```python
from build123d import *

# Parameters (mm, degrees)
SKETCH1_R           = 4.5
SKETCH1_R_2         = 2.55
BOSS_EXTRUDE1_DEPTH = 3
SKETCH2_R           = 2.55
BOSS_EXTRUDE2_DEPTH = 4
CHAMFER1_SIZE       = 2
CUT_EXTRUDE1_DEPTH  = 32.132780152
BOSS_EXTRUDE4_DEPTH = 5
CHAMFER2_SIZE       = 1


with BuildPart() as part:
    # Sketch1 → Boss-Extrude1 (new body)
    with BuildSketch(Plane(origin=(0, 0, 0), x_dir=(1, 0, 0), z_dir=(0, 1, 0))):
        with Locations(Location((0, 0, 0), (0, 0, 270))):
            Circle(SKETCH1_R)
        with Locations(Location((0, 0, 0), (0, 0, 270))):
            Circle(SKETCH1_R_2, mode=Mode.SUBTRACT)
    extrude(amount=BOSS_EXTRUDE1_DEPTH)

    # Sketch2 → Boss-Extrude2 (add)
    with BuildSketch(Plane(origin=(0, 3, 0), x_dir=(1, 0, 0), z_dir=(0, 1, 0))):
        with BuildLine():
            Line((0, -4.5), (30, -4.5))
            Line((30, -4.5), (30, 4.5))
            Line((30, 4.5), (0, 4.5))
            ThreePointArc((0, 4.5), (-4.5, 0), (0, -4.5))
        make_face()
        with Locations(Location((0, 0, 0), (0, 0, 270))):
            Circle(SKETCH2_R, mode=Mode.SUBTRACT)
    extrude(amount=BOSS_EXTRUDE2_DEPTH)

    # Chamfer1
    # the kernel refuses this chamfer: 2 mm, written as the material it takes off along each edge
    with BuildSketch(Plane(origin=(28.666666667, 4.333333333, 3.166666667), x_dir=(-0.7071067811865475, -0.7071067811865475, 0), z_dir=(0.5773502691896256, -0.5773502691896258, 0.5773502691896258))) as chamfer1_piece_1:
        Polygon((-1.414213562, 0.816496581), (1.414213562, 0.816496581), (0, -1.632993162), align=None)
    extrude(amount=2.540341184, mode=Mode.SUBTRACT)
    with BuildSketch(Plane(origin=(28.666666667, 4.333333333, -3.166666667), x_dir=(-0.7071067811865476, -0.7071067811865475, 0), z_dir=(0.5773502691896256, -0.5773502691896258, -0.5773502691896257))) as chamfer1_piece_2:
        Polygon((-1.414213562, -0.816496581), (1.414213562, -0.816496581), (0, 1.632993162), align=None)
    extrude(amount=2.540341184, mode=Mode.SUBTRACT)
    with BuildSketch(Plane(origin=(-5.143365976, 3, 4.5), x_dir=(0, -0.027495876610586275, -0.9996219169112968), z_dir=(1, 0, 0))) as chamfer1_piece_3_section:
        Polygon((CHAMFER1_SIZE * 0.999621916911, CHAMFER1_SIZE * 0.0274958766106), (-CHAMFER1_SIZE * 0.0274958766106, CHAMFER1_SIZE * 0.999621916911), (0, 0), align=None)
    chamfer1_piece_3 = extrude(amount=40.286731952, mode=Mode.PRIVATE)
    chamfer1_piece_3 = chamfer1_piece_3 - Plane(origin=(0, 3.673505516, 0), x_dir=(0, 0, 1), z_dir=(0, -1, 0)) * Cylinder(4.5, 89, mode=Mode.PRIVATE)
    add(chamfer1_piece_3, mode=Mode.SUBTRACT)
    with BuildSketch(Plane(origin=(30, 3, 9.643365976), x_dir=(-0.9996219169112968, -0.027495876610586296, 0), z_dir=(0, 0, -1))) as chamfer1_piece_4:
        Polygon((CHAMFER1_SIZE * 0.999621916911, CHAMFER1_SIZE * 0.0274958766106), (-CHAMFER1_SIZE * 0.0274958766106, CHAMFER1_SIZE * 0.999621916911), (0, 0), align=None)
    extrude(amount=19.286731952, mode=Mode.SUBTRACT)
    with BuildSketch(Plane(origin=(30, -2.143365976, 4.5), x_dir=(-0.9996219169112968, 0, 0.02749587661058651), z_dir=(0, 1, 0))) as chamfer1_piece_5:
        Polygon((CHAMFER1_SIZE * 0.999621916911, -CHAMFER1_SIZE * 0.0274958766106), (-CHAMFER1_SIZE * 0.0274958766106, -CHAMFER1_SIZE * 0.999621916911), (0, 0), align=None)
    extrude(amount=14.286731952, mode=Mode.SUBTRACT)
    with BuildSketch(Plane(origin=(35.143365976, 3, -4.5), x_dir=(0, -0.027495876610586275, 0.9996219169112968), z_dir=(-1, 0, 0))) as chamfer1_piece_6_section:
        Polygon((CHAMFER1_SIZE * 0.999621916911, CHAMFER1_SIZE * 0.0274958766106), (-CHAMFER1_SIZE * 0.0274958766106, CHAMFER1_SIZE * 0.999621916911), (0, 0), align=None)
    chamfer1_piece_6 = extrude(amount=40.286731952, mode=Mode.PRIVATE)
    chamfer1_piece_6 = chamfer1_piece_6 - Plane(origin=(0, 3.673505518, 0), x_dir=(0, 0, 1), z_dir=(0, -1, 0)) * Cylinder(4.5, 89, mode=Mode.PRIVATE)
    add(chamfer1_piece_6, mode=Mode.SUBTRACT)
    with BuildSketch(Plane(origin=(30, -2.143365976, -4.5), x_dir=(-0.9996219169112968, 0, -0.02749587661058651), z_dir=(0, 1, 0))) as chamfer1_piece_7:
        Polygon((CHAMFER1_SIZE * 0.999621916911, CHAMFER1_SIZE * 0.0274958766106), (-CHAMFER1_SIZE * 0.0274958766106, CHAMFER1_SIZE * 0.999621916911), (0, 0), align=None)
    extrude(amount=14.286731952, mode=Mode.SUBTRACT)

    # Sketch3 → Cut-Extrude1 (cut, through all)
    with BuildSketch(Plane(origin=(0, 7, 0), x_dir=(1, 0, 0), z_dir=(0, 1, 0))):
        Polygon((18, 1.3), (18, -1.3), (30, -1.3), (30, 2.5), (28, 4.5), (18, 4.5), align=None)
    extrude(amount=-CUT_EXTRUDE1_DEPTH, mode=Mode.SUBTRACT)

    # Sketch3<4> → Boss-Extrude4 (add)
    with BuildSketch(Plane(origin=(0, 7, 0), x_dir=(1, 0, 0), z_dir=(0, 1, 0))):
        Polygon((5.4, 3.25), (5.4, -3.25), (7.4, -3.25), (7.4, -1.3), (18, -1.3), (18, 1.3), (7.4, 1.3), (7.4, 3.25), align=None)
    extrude(amount=BOSS_EXTRUDE4_DEPTH)

    # Chamfer2
    chamfer2_edges = [part.edges().sort_by_distance(p)[0] for p in [
        (29, 4, 1.3),
        (18, 4, -3.5),
        (18, 5, 1.3),
        (30, 6, 1.3),
        (23, 3, 1.3),
        (18, 3, -0.6),
        (18, 6, -4.5),
    ]]
    chamfer(chamfer2_edges, length=CHAMFER2_SIZE)


solid = part.part
```
Source: CAD feature listing. Evaluate the final solid. Frame: model axes, mm. A direction names the side the tool comes from. Give positions to 0.01 mm unless a question says otherwise; leave off trailing zeros. Loops run counter-clockwise (first coordinate to the right, second up) from the corner with the lowest first, then second, coordinate; pieces in that order, holes last. Notation, with made-up numbers: M -7,37.5 L 14,37.5 A20 cw 14,72.5 Z; hole C 86,21 d6. An arc over 180 degrees is marked long. Put each result on its own line as item: value.
Q1. Section B-B (z = -1.75). Return the cut outline in (x, y), and give its area (3 significant figures).
Response values:
outline: M -4.15,0 L -1.85,0 L -1.85,7 L -4.15,7 Z; M 1.85,0 L 4.15,0 L 4.15,3 L 17,3 L 18,4 L 18,7 L 7.4,7 L 7.4,12 L 5.4,12 L 5.4,7 L 1.85,7 Z
area: 97.0 mm²
Q2. Section C-C (x = 25). Return the cut outline in (y, z), and give its area (3 significant figures).
Response values:
outline: M 3,2.3 L 4,1.3 L 7,1.3 L 7,4.5 L 5,4.5 L 3,2.5 Z
area: 10.3 mm²
Q3. Reachability of faces 1 (the flat face through (24, 6, 1.3)), 2 (the flat face through (13.8, 4, 3.5)), 3 (the flat face through (5.4, 9, 0)), 4 (the cylindrical face through (-4.49, 3.45, -0.3)), 5 (the flat face through (23.4, 3.5, 1.8)) from +Z, -Z, +X, -X, +Y, -Y: full face, straight path, thin tool, end or side. Return the list, or none.
Response values:
face 1: -Z, +X, +Y, -Y
face 2: +Z, +X, -Y
face 3: +Z, -Z, -X, +Y
face 4: -Y
face 5: -Z, +X, -Y
Q4. Line query: probe 1 along Y at (x, z) = (16.5, -1); probe 2 along X at (y, z) = (11, -1); probe 3 along Z at (x, y) = (1.5, 4.5). Output: solid intervals per line, ascending. Write a range as [from, to].
Response values:
probe 1: y = [3, 12]
probe 2: x = [5.4, 18]
probe 3: z = [-4.24, -2.06], [2.06, 4.24]
Q5. Pin query (flat end, axial travel): P1, Ø4, axis at x = 14, y = 10.5, coming from the -Z side; P2, Ø0.6, axis at y = 10, z = 2, coming from the +X side; P3, Ø1.5, axis at y = 1, z = 2.5, coming from the -X side; P4, Ø3, axis at x = 3, y = 9, coming from the +Z side. Return the tip coordinate at first contact, or that it passes through.
Response values:
P1: stops at z = -1.3
P2: stops at x = 7.4
P3: stops at x = -4.15
P4: passes through
Q6. Section A-A (y = 6.5). Return the cut outline in (x, z).
Response values:
outline: M 0,-4.5 L 17,-4.5 L 18,-3.5 L 18,0.3 L 19,1.3 L 29,1.3 L 30,2.3 L 30,2.5 L 28,4.5 L 0,4.5 A4.5 ccw Z; hole C 0,0 d5.1
Q7. Section D-D (y = 2.5). Return the cut outline in (x, z).
Response values:
outline: C 0,0 d9; hole C 0,0 d5.1
